Part model, mm, in its own coordinate system. A direction names the side the tool comes from. Round coordinates to 2 decimals unless told otherwise and drop trailing zeros. Write each loop counter-clockwise with the first axis right and the second up, starting at its lowest first coordinate (ties: lowest second). Pieces come first, ordered by that corner, then holes. Notation, with made-up numbers: M 54,-25.5 L 67,-25.5 A13 ccw 67,-0.5 Z; hole C 12,-36 d11. An arc over 180 degrees is marked long. One line per question, with ' | ' between items. Start each with the question number.
1) Saw through at B-B (x = 16.5). List the corners of the cut face in (y, z), plus the area to 3 significant figures.
2) Drop flat-ended pins along their axis: pin 1 Ø8 at (x, z) = (5.5, 0) entering from +Y; pin 2 Ø8 at (x, z) = (14.5, -18) entering from +Y; pin 3 Ø5 at (y, z) = (40.5, 17.5) entering from +X. Give the stop position or say it passes through.
3) Saw through at A-A (z = -19.5). List the corners of the cut face in (x, y) (1 decimal), plus the area to 3 significant figures.
4) Tool access for faces 1 (the face through (4.6, 16.1, -50)), 2 (the face through (4.762, 29, -1)): list every direction of +Z, -Z, +X, -X, +Y, -Y with a clear straight run to the whole face (end or side of a thin tool).
5) Wall check: probe 1 along X at (y, z) = (12.5, -26.5); probe 2 along X at (y, z) = (3.5, -8.5). Give the ranges that are in metal, low to high. Write a range as [from, to].
Autodesk Inventor part; units mm, degrees
ref_plane "YZ Plane" through (0, 0, 0) normal (1, 0, 0) x (0, 1, 0)
ref_plane "XZ Plane" through (0, 0, 0) normal (0, 1, 0) x (-1, 0, 0)
ref_plane "XY Plane" through (0, 0, 0) normal (0, 0, 1) x (1, 0, 0)
sketch "Sketch1" plane through (0, 0, 0) normal (0, 0, 1) x (1, 0, 0)
  line L0 (0, 0) -> (0, 50.8)
  line L1 (0, 50.8) -> (1.524, 50.8)
  line L2 (4.7625, 47.5615) -> (4.7625, 9.525)
  line L3 (0, 0) -> (50.8, 0)
  line L4 (50.8, 0) -> (50.8, 1.524)
  line L5 (47.5615, 4.7625) -> (9.525, 4.7625)
  arc A0 (4.7625, 9.525) -> (9.525, 4.7625) centre (9.525, 9.525) ccw
  arc A1 (4.7625, 47.5615) -> (1.524, 50.8) centre (1.524, 47.5615) ccw
  arc A2 (50.8, 1.524) -> (47.5615, 4.7625) centre (47.5615, 1.524) ccw
  dimension "thickness" = 4.7625
  dimension "d3" = 4.7625
  dimension "LegSize" = 50.8
  dimension "d5" = 50.8
  dimension "radius" = 4.7625
  dimension "d7" = 3.2385
  dimension "d8" = 3.2385
extrude "2\" X 2\" X 3/16\"" add sketch "Sketch1" along normal mid plane 100
equation "\"d3\" = thickness"
equation "\"d5\" = LegSize"
properties part number "ANGLE IRON, 2 X 2 X 0.188 THK" material "Angle Iron"
Answer key:
1) outline: M 0,-50 L 4.76,-50 L 4.76,50 L 0,50 Z | area: 476 mm2
2) pin 1: stops at y = 50.8 | pin 2: stops at y = 4.76 | pin 3: stops at x = 4.76
3) outline: M 0,0 L 50.8,0 L 50.8,1.5 A3.2 ccw 47.6,4.8 L 9.5,4.8 A4.8 cw 4.8,9.5 L 4.8,47.6 A3.2 ccw 1.5,50.8 L 0,50.8 Z | area: 462 mm2
4) face 1: -Z, +X, -X, +Y, -Y | face 2: +Z, -Z, +X, +Y
5) probe 1: x = [0, 4.76] | probe 2: x = [0, 50.13]
